from build123d import *

# Parameters (mm, degrees)
SKETCH_1_R          = 10
SKETCH_1_R_2        = 2.55
EXTRUDE_1_DEPTH     = 15
SKETCH_3_R          = 1.6
CUT_EXTRUDE_1_DEPTH = 21
EXTRUDE_2_DEPTH     = 6
SKETCH_6_R          = 2.55
CUT_EXTRUDE_2_DEPTH = 10
SKETCH_7_W          = 40
SKETCH_7_H          = 42
EXTRUDE_3_DEPTH     = 6
SKETCH_8_R          = 1.6
CUT_EXTRUDE_3_DEPTH = 6
SKETCH_9_W          = 46
SKETCH_9_H          = 2
EXTRUDE_4_DEPTH     = 19
SKETCH_10_R         = 13
CUT_EXTRUDE_4_DEPTH = 8
SKETCH_11_W         = 8
SKETCH_11_H         = 15
CUT_EXTRUDE_5_DEPTH = 8


with BuildPart() as part:
    # 草图1 → 凸台-拉伸1 (new body)
    with BuildSketch(Plane.XY):
        with Locations((-2.14168272, 2.06384273)):
            Circle(SKETCH_1_R)
        with Locations((-2.14168272, 2.06384273)):
            Circle(SKETCH_1_R_2, mode=Mode.SUBTRACT)
    extrude(amount=EXTRUDE_1_DEPTH)

    # 草图3 → 切除-拉伸1 (cut, through all)
    with BuildSketch(Plane(origin=(7.85831728, 0, 0), x_dir=(0, 0, -1), z_dir=(1, 0, 0))):
        with Locations((-7.5, 2.06384273)):
            Circle(SKETCH_3_R)
    extrude(amount=-CUT_EXTRUDE_1_DEPTH, mode=Mode.SUBTRACT)

    # 草图5 → 凸台-拉伸2 (add)
    with BuildSketch(Plane.XY.offset(15)):
        with BuildLine():
            Line((-2.14168272, 23.06384273), (32.85831728, 23.06384273))
            Line((32.85831728, 23.06384273), (32.85831728, -18.93615727))
            Line((32.85831728, -18.93615727), (-2.14168272, -18.93615727))
            ThreePointArc((-2.14168272, -18.93615727), (-23.14168272, 2.06384273), (-2.14168272, 23.06384273))
        make_face()
    extrude(amount=EXTRUDE_2_DEPTH)

    # 草图6 → 切除-拉伸2 (cut)
    with BuildSketch(Plane(origin=(0, 0, 15), x_dir=(-1, 0, 0), z_dir=(0, 0, -1))):
        with Locations((2.14168272, 2.06384273)):
            Circle(SKETCH_6_R)
    extrude(amount=-CUT_EXTRUDE_2_DEPTH, mode=Mode.SUBTRACT)

    # 草图7 → 凸台-拉伸3 (add)
    with BuildSketch(Plane(origin=(32.85831728, 0, 0), x_dir=(0, 0, -1), z_dir=(1, 0, 0))):
        with Locations((5, 2.06384273)):
            Rectangle(SKETCH_7_W, SKETCH_7_H)
    extrude(amount=-EXTRUDE_3_DEPTH)

    # 草图8 → 切除-拉伸3 (cut)
    with BuildSketch(Plane(origin=(32.85831728, 0, 0), x_dir=(0, 0, -1), z_dir=(1, 0, 0))):
        with Locations((0, 19.06384273)):
            Circle(SKETCH_8_R)
        with Locations((0, -14.93615727)):
            Circle(SKETCH_8_R)
        with Locations((20, -14.93615727)):
            Circle(SKETCH_8_R)
        with Locations((20, 19.06384273)):
            Circle(SKETCH_8_R)
    extrude(amount=-CUT_EXTRUDE_3_DEPTH, mode=Mode.SUBTRACT)

    # 草图9 → 凸台-拉伸4 (add)
    with BuildSketch(Plane(origin=(32.85831728, 0, 0), x_dir=(0, 0, -1), z_dir=(1, 0, 0))):
        with Locations((2, 10.61384273)):
            Rectangle(SKETCH_9_W, SKETCH_9_H)
        with Locations((2, -6.48615727)):
            Rectangle(SKETCH_9_W, SKETCH_9_H)
    extrude(amount=EXTRUDE_4_DEPTH)

    # 草图10 → 切除-拉伸4 (cut)
    with BuildSketch(Plane.XZ.offset(7.48615727)):
        with Locations((51.85831728, -2)):
            Circle(SKETCH_10_R)
    extrude(amount=-CUT_EXTRUDE_4_DEPTH, mode=Mode.SUBTRACT)

    # 草图11 → 切除-拉伸5 (cut)
    with BuildSketch(Plane(origin=(0, 11.61384273, 0), x_dir=(1, 0, 0), z_dir=(0, 1, 0))):
        with Locations((39.85831728, -3.5)):
            Rectangle(SKETCH_11_W, SKETCH_11_H)
    extrude(amount=-CUT_EXTRUDE_5_DEPTH, mode=Mode.SUBTRACT)


solid = part.part
Could you check a few things on this model? Use its own coordinates, in mm. A direction names the side the tool comes from. Round coordinates to 2 decimals unless told otherwise and drop trailing zeros. Order: outer loops, then holes, each group sorted by start corner. A loop starts at its lowest first (then second) coordinate and runs counter-clockwise, first axis right, second up.
(1) Please list where these lines run through material, in increasing order: line 1 along Y through (x, z) = (35, 5); line 2 along X through (y, z) = (1.5, -6); line 3 along Y through (x, z) = (-6.75, 7.5).
Response values:
line 1: y = -7.49 to -5.49, 9.61 to 11.61
line 2: x = 26.86 to 32.86
line 3: y = -6.81 to 0.46, 3.66 to 10.94
(2) Which directions (+Z, -Z, +X, -X, +Y, -Y) give clear straight access to the entire face, cutting with the end or side of a thin tool? Please do faces 1 (the flat face through (32.858, -13, -2)), 2 (the cylindrical face through (3.907, 0.502, 7.847)), 3 (the flat face through (44.3, 11.614, -1.7)).
Response values:
face 1: +Z, -Z, +X, -Y
face 2: -X
face 3: +Z, -Z, +X, +Y
(3) Imagine slicing it at C-C (y = 10.5). Write out the boundary of the cut face in (x, z), plus the area to 3 significant figures.
Response values:
outline: (-21.37, 15) - (-7.51, 15) - (-7.51, 0) - (3.23, 0) - (3.23, 15) - (26.86, 15) - (26.86, -25) - (51.86, -25) - (51.86, 21) - (-21.37, 21) - close; hole (35.86, -4) - (43.86, -4) - (43.86, 11) - (35.86, 11) - close
area: 1,480 mm2
(4) I'm going to push flat-ended pins straight in: pin 1 (2 mm diameter, centred on y = 10.5, z = 6, fed in from -X); pin 2 (4 mm diameter, centred on y = 2.06, z = 7.5, fed in from +X); pin 3 (12 mm diameter, centred on y = -1, z = -10.5, fed in from -X). Where does each tip first touch, or does it pass through?
Response values:
pin 1: stops at x = -8.83
pin 2: stops at x = 32.86
pin 3: stops at x = 26.86
(5) Imagine slicing it at D-D (x = 7). Write out the boundary of the cut face in (y, z).
Response values:
outline: (-18.94, 15) - (-1.99, 15) - (-1.99, 0) - (6.12, 0) - (6.12, 15) - (23.06, 15) - (23.06, 21) - (-18.94, 21) - close; hole circle Ø3.2 at (2.06, 7.5)
(6) Imagine slicing it at A-A (z = -20). Write out the boundary of the cut face in (x, y), plus the area to 3 significant figures.
Response values:
outline: (26.86, -18.94) - (32.86, -18.94) - (32.86, -16.54) - (26.86, -16.54) - close; (26.86, -13.34) - (32.86, -13.34) - (32.86, -7.49) - (51.86, -7.49) - (51.86, -5.49) - (32.86, -5.49) - (32.86, 9.61) - (51.86, 9.61) - (51.86, 11.61) - (32.86, 11.61) - (32.86, 17.46) - (26.86, 17.46) - close; (26.86, 20.66) - (32.86, 20.66) - (32.86, 23.06) - (26.86, 23.06) - close
area: 290 mm2
(7) Imagine slicing it at B-B (z = 12). Write out the boundary of the cut face in (x, y), plus the area to 3 significant figures.
Response values:
outline: circle Ø20 at (-2.14, 2.06); (26.86, -18.94) - (32.86, -18.94) - (32.86, -7.49) - (51.86, -7.49) - (51.86, -5.49) - (32.86, -5.49) - (32.86, 9.61) - (51.86, 9.61) - (51.86, 11.61) - (32.86, 11.61) - (32.86, 23.06) - (26.86, 23.06) - close; hole circle Ø5.1 at (-2.14, 2.06)
area: 622 mm2
(8) If we mould it in two halves opening along Z, with no side actions, what happens to faces 4 (the flat face through (31, 0, -25)), 5 (the flat face through (40, 11, 11)), 6 (the cylindrical face through (29.9, -15.91, -18.73)), 7 (the flat face through (38, -5.486, -2))? For each: released by +Z, released by -Z, zero draft, split by the parting line, or undercut.
Response values:
face 4: released by -Z
face 5: undercut
face 6: undercut
face 7: zero draft
